For this review, take the finished solid that the model builds, in its own axes (mm). A direction names the side the tool comes from. Round coordinates to 2 decimals unless told otherwise and drop trailing zeros. Order: outer loops, then holes, each group sorted by start corner. A loop starts at its lowest first (then second) coordinate and runs counter-clockwise, first axis right, second up.
```python
from build123d import *

# Parameters (mm, degrees)
SKETCH3_W               = 19.05
SKETCH3_H               = 19.05
BOSS_EXTRUDE1_DEPTH     = 100
SKETCH5_W               = 16.65
SKETCH5_H               = 16.65
CUT_EXTRUDE1_DEPTH      = 201.453114842
CUT_EXTRUDE2_DEPTH      = 101.903177601
CUT_EXTRUDE2_DEPTH_BACK = 101.903177601


with BuildPart() as part:
    # Sketch3 → Boss-Extrude1 (new, symmetric)
    with BuildSketch(Plane.XY):
        Rectangle(SKETCH3_W, SKETCH3_H)
    extrude(amount=BOSS_EXTRUDE1_DEPTH, both=True)

    # Sketch5 → Cut-Extrude1 (cut, through all)
    with BuildSketch(Plane(origin=(0, 0, -100), x_dir=(-1, 0, 0), z_dir=(0, 0, -1))):
        Rectangle(SKETCH5_W, SKETCH5_H)
    extrude(amount=-CUT_EXTRUDE1_DEPTH, mode=Mode.SUBTRACT)

    # Sketch7 → Cut-Extrude2 (cut, two sides: drawn at the far end of the back side and taken through both)
    with BuildSketch(Plane(origin=(0, 0, 0), x_dir=(1, 0, 0), z_dir=(0, 1, 0)).offset(-CUT_EXTRUDE2_DEPTH_BACK)):
        Polygon((9.525, 100), (-9.525, 100), (-9.525, 80.95), align=None)
        Polygon((-9.525, -80.95), (9.525, -100), (-9.525, -100), align=None)
    extrude(amount=CUT_EXTRUDE2_DEPTH + CUT_EXTRUDE2_DEPTH_BACK, mode=Mode.SUBTRACT)


solid = part.part
```
Q1. Tool access review of faces 1 (the face through (0, 9.525, 1)), 2 (the face through (0, -8.325, -1)): name each direction out of +Z, -Z, +X, -X, +Y, -Y from which nothing blocks a thin tool from reaching the whole face with its end or side.
Q2. Wall thickness on line 1 (Y direction, x = -4, z = -45) (3 decimals); line 2 (X direction, y = 6.25, z = -85) (3 decimals): over which ranges is each line inside the solid? List them lowest first.
Q3. Take a section at C-C, the plane x = 5.5. State the section outline as (y, z) points (3 decimals), plus the area to 3 significant figures.
Q4. Take a section at A-A, the plane y = 2.5. State the section outline as (x, z) points (3 decimals), plus the area to 3 significant figures.
Q5. Take a section at B-B, the plane z = -45. State the section outline as (x, y) points (3 decimals).
Q6. Mouldability with a two-part tool opening along Y and no side actions: class faces 3 (the face through (8.325, 0, -1)), 4 (the face through (-9.525, 0, 1)), 5 (the face through (0, -9.525, 1)), 6 (the face through (-8.325, 0, -1)) as +Y half, -Y half, draft (parallel to the pull), parting line (faces both ways), or undercut.
Working result:
1. face 1: +Z, -Z, +X, -X, +Y
1. face 2: +Z, -Z
2. line 1: y = -9.525 to -8.325, 8.325 to 9.525
2. line 2: x = 8.325 to 9.525
3. outline: (-9.525, -95.975) - (-8.325, -95.975) - (-8.325, 95.975) - (-9.525, 95.975) - close; (8.325, -95.975) - (9.525, -95.975) - (9.525, 95.975) - (8.325, 95.975) - close
3. area: 461 mm2
4. outline: (-9.525, -80.95) - (-8.325, -82.15) - (-8.325, 82.15) - (-9.525, 80.95) - close; (8.325, -98.8) - (9.525, -100) - (9.525, 100) - (8.325, 98.8) - close
4. area: 434 mm2
5. outline: (-9.525, -9.525) - (9.525, -9.525) - (9.525, 9.525) - (-9.525, 9.525) - close; hole (-8.325, -8.325) - (8.325, -8.325) - (8.325, 8.325) - (-8.325, 8.325) - close
6. face 3: undercut
6. face 4: draft
6. face 5: -Y half
6. face 6: undercut
